Verification items for the finished model (mm, model axes). Face numbers are marked on the shaded views. A direction names the side the tool comes from. Give positions to 0.01 mm unless a question says otherwise; leave off trailing zeros. Order: outer loops, then holes, each group sorted by start corner. A loop starts at its lowest first (then second) coordinate and runs counter-clockwise, first axis right, second up. Notation, with made-up numbers: M 23.25,-32.75 L 53.25,-32.75 A11 cw 53.25,-23.75 Z; hole C 37.5,-28 d8. An arc over 180 degrees is marked long. Answer as a JSON object with one key per item and string values.
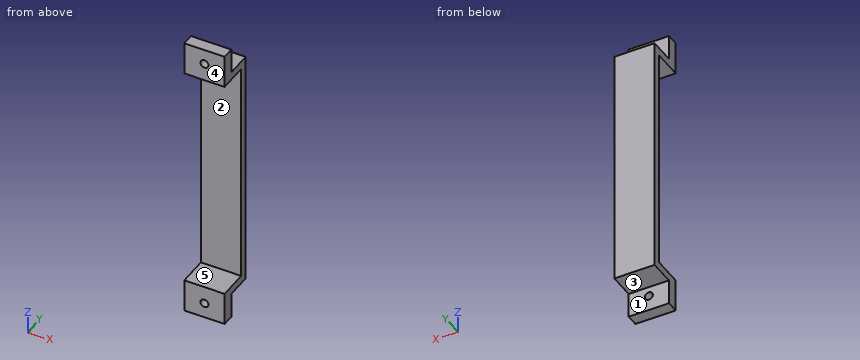
```python
from build123d import *

# Parameters (mm, degrees)
SKETCH_1_W      = 5
SKETCH_1_H      = 3.09
SKETCH_1_R      = 0.5
SKETCH_1_H_2    = 1
EXTRUDE_1_DEPTH = 1.5
SKETCH_1_3_W    = 5
SKETCH_1_3_H    = 1
EXTRUDE_2_DEPTH = 3.7
SKETCH_2_W      = 5
SKETCH_2_H      = 15.05
EXTRUDE_3_DEPTH = 1


with BuildPart() as part:
    # Sketch 1 → Extrude 1 (new body)
    # profile 1 of 2: a face of its own
    with BuildSketch(Plane(origin=(0, 0, 0), x_dir=(1, 0, 0), z_dir=(0, 1, 0))):
        with Locations((2.5, -1.545)):
            Rectangle(SKETCH_1_W, SKETCH_1_H)
        with Locations(Location((2.5, -1.89, 0), (0, 0, 270))):
            Circle(SKETCH_1_R, mode=Mode.SUBTRACT)
    # profile 2 of 2: a face of its own
    with BuildSketch(Plane(origin=(0, 0, 0), x_dir=(1, 0, 0), z_dir=(0, 1, 0))):
        with Locations((2.5, -3.59)):
            Rectangle(SKETCH_1_W, SKETCH_1_H_2)
    extrude_1 = extrude(amount=EXTRUDE_1_DEPTH)

    # Sketch 1_3 → Extrude 2 (add)
    with BuildSketch(Plane(origin=(0, 0, 0), x_dir=(1, 0, 0), z_dir=(0, 1, 0))):
        with Locations((2.5, -3.59)):
            Rectangle(SKETCH_1_3_W, SKETCH_1_3_H)
    extrude_2 = extrude(amount=EXTRUDE_2_DEPTH)

    # Sketch 2 → Extrude 3 (add)
    with BuildSketch(Plane(origin=(0, 3.7, 0), x_dir=(1, 0, 0), z_dir=(0, 1, 0))):
        with Locations((2.5, -10.615)):
            Rectangle(SKETCH_2_W, SKETCH_2_H)
    extrude_3 = extrude(amount=EXTRUDE_3_DEPTH)

    # Mirror 1: Extrude 1, Extrude 2, Extrude 3 across plane
    add(extrude_1.mirror(Plane(origin=(0, 4.7, 18.14), x_dir=(1, 0, 0), z_dir=(0, 0, -1))))
    add(extrude_2.mirror(Plane(origin=(0, 4.7, 18.14), x_dir=(1, 0, 0), z_dir=(0, 0, -1))))
    add(extrude_3.mirror(Plane(origin=(0, 4.7, 18.14), x_dir=(1, 0, 0), z_dir=(0, 0, -1))))


solid = part.part
```
Q1. Section check B-B on y = 0.65. Record the cut outline in (x, z), then the cut area to 3 significant figures.
Resolved:
{"outline": "M 0,0 L 5,0 L 5,4.09 L 0,4.09 Z; M 0,32.19 L 5,32.19 L 5,36.28 L 0,36.28 Z; hole C 2.5,1.89 d1; hole C 2.5,34.39 d1", "area": "39.3 mm²"}
Q2. Tool access check on the marked faces 4 and 5. Record the directions out of +Z, -Z, +X, -X, +Y, -Y that give a thin tool (end or side, any length) a straight path to the whole face; none if there is none.
Resolved:
{"face 4": "+Z, -Z, +X, -X, -Y", "face 5": "+X, -X, -Y"}
Q3. Section check D-D on y = 2.8. Record the cut outline in (x, z).
Resolved:
{"outline": "M 0,3.09 L 5,3.09 L 5,4.09 L 0,4.09 Z; M 0,32.19 L 5,32.19 L 5,33.19 L 0,33.19 Z"}
Q4. Section check C-C on x = 2.5. Record the cut outline in (y, z), then the cut area to 3 significant figures.
Resolved:
{"outline": "M 0,0 L 1.5,0 L 1.5,1.39 L 0,1.39 Z; M 0,2.39 L 1.5,2.39 L 1.5,3.09 L 4.7,3.09 L 4.7,33.19 L 1.5,33.19 L 1.5,33.89 L 0,33.89 L 0,32.19 L 3.7,32.19 L 3.7,4.09 L 0,4.09 Z; M 0,34.89 L 1.5,34.89 L 1.5,36.28 L 0,36.28 Z", "area": "43.8 mm²"}
Q5. Release check for a two-part mould opening along Z. For the marked faces 1, 2 and 3 record: +Z half, -Z half, draft (parallel to the pull), parting line (faces both ways), or undercut.
Resolved:
{"face 1": "draft", "face 2": "undercut", "face 3": "-Z half"}
Q6. Material ranges on L1, parallel to Z at x = 2.5, y = 3.6; L2, parallel to X at y = 0.85, z = 1.89; L3, parallel to Z at x = 3.1, y = 1, recorded low to high.
Resolved:
{"L1": "z = 3.09 to 4.09, 32.19 to 33.19", "L2": "x = 0 to 2, 3 to 5", "L3": "z = 0 to 4.09, 32.19 to 36.28"}
Q7. Section check A-A on z = 34.39. Record the cut outline in (x, y).
Resolved:
{"outline": "M 0,0 L 2,0 L 2,1.5 L 0,1.5 Z; M 3,0 L 5,0 L 5,1.5 L 3,1.5 Z"}
Q8. Gauge pin test, flat ends, axial feed: pin 1 Ø2.5 at (x, z) = (3, 2) entering from +Y; pin 2 Ø3 at (x, z) = (3.5, 19) entering from -Y; pin 3 Ø1 at (x, y) = (2, 3) entering from -Z; pin 4 Ø2.5 at (x, z) = (3.5, 34.5) entering from +Y. Record the tip position at first contact, or that the pin passes through.
Resolved:
{"pin 1": "stops at y = 4.7", "pin 2": "stops at y = 3.7", "pin 3": "stops at z = 3.09", "pin 4": "stops at y = 1.5"}
